Source: CAD feature listing. Evaluate the final solid. Frame: model axes, mm. A direction names the side the tool comes from. Coordinates: 2 decimals unless noted, no trailing zeros. Write each loop counter-clockwise with the first axis right and the second up, starting at its lowest first coordinate (ties: lowest second). Pieces come first, ordered by that corner, then holes. Notation, with made-up numbers: M -22.5,-23.75 L 25.5,-23.75 A34 ccw 25.5,9.25 Z; hole C 29,19 d1. An arc over 180 degrees is marked long. One line per item, written item: value. Start each with the question number.
Item 1: Set-up query: faces 1 (the flat face through (-29, 0, -7.845)), 2 (the flat face through (-3, -16.25, 11)), 3 (the flat face through (16, 27.428, 5)). Return all of +Z, -Z, +X, -X, +Y, -Y with unobstructed straight access to the full face (end or side cutting, diameter ignored); none if empty.
Item 2: Ray query, L1, parallel to X at y = -26.5, z = 9.5; L2, parallel to Y at x = -22.5, z = 8.75; L3, parallel to X at y = -12, z = 7.75. Return the intervals inside material, ascending. Write a range as from..to.
Item 3: Cut plane C-C, the plane y = 9. Output: boundary loops of the cut face in (x, z), then the cut area to 3 significant figures.
Item 4: Cut plane D-D, the plane z = -6. Output: boundary loops of the cut face in (x, y).
Item 5: Pin query (flat end, axial travel): P1, Ø5, axis at x = -8.5, z = -4.5, coming from the -Y side; P2, Ø5, axis at x = 1.5, z = -4, coming from the -Y side; P3, Ø3, axis at x = -27.5, z = -4.5, coming from the +Y side; P4, Ø1.8, axis at y = -1.5, z = -3.5, coming from the +X side. Return the tip coordinate at first contact, or that it passes through.
Item 6: Cut plane B-B, the plane z = 5.5. Output: boundary loops of the cut face in (x, y), then the cut area to 3 significant figures.
Item 7: Mould query, pull axis X, two halves, no side actions, for faces 4 (the flat face through (-28.664, -0.208, -9.431)), 5 (the flat face through (0, 27.428, -4)), 6 (the flat face through (-16, -27.928, 5)). Classes: released by +X, released by -X, zero draft, split by the parting line, or undercut.
Item 8: Cut plane A-A, the plane x = 4. Output: boundary loops of the cut face in (y, z), then the cut area to 3 significant figures.
Autodesk Inventor part; units mm, degrees
ref_plane "YZ Plane" through (0, 0, 0) normal (1, 0, 0) x (0, 1, 0)
ref_plane "XZ Plane" through (0, 0, 0) normal (0, 1, 0) x (-1, 0, 0)
ref_plane "XY Plane" through (0, 0, 0) normal (0, 0, 1) x (1, 0, 0)
sketch "Эскиз1" plane through (0, 0, 0) normal (0, 0, 1) x (1, 0, 0)
  line L0 (41.178, 40.928) -> (-41.178, 40.928) construction
  line L1 (-41.178, 40.928) -> (-41.178, -40.928) construction
  line L2 (-41.178, -40.928) -> (41.178, -40.928) construction
  line L3 (41.178, -40.928) -> (41.178, 40.928) construction
  circle A0 centre (22.7283, 19.0964) radius 1 construction
  circle A1 centre (19.3464, -22.9783) radius 1 construction
  line L4 (17.2251, 27.428) -> (22.7282, 21.9249) construction
  line L5 (22.7282, 21.9249) -> (19.8998, 19.0964) construction
  line L6 (19.8998, 19.0964) -> (22.7282, 16.268) construction
  line L7 (22.7282, 16.268) -> (25.5567, 19.0964) construction
  line L8 (25.5567, 19.0964) -> (27.678, 16.9751) construction
  line L9 (27.678, 16.9751) -> (27.678, -17.4751) construction
  line L10 (27.678, -17.4751) -> (22.1749, -22.9783) construction
  line L11 (22.1749, -22.9783) -> (19.3464, -20.1498) construction
  line L12 (19.3464, -20.1498) -> (16.518, -22.9783) construction
  line L13 (16.518, -22.9783) -> (19.3464, -25.8067) construction
  line L14 (19.3464, -25.8067) -> (17.2251, -27.928) construction
  line L15 (17.2251, -27.928) -> (-17.2251, -27.928) construction
  line L16 (-17.2251, -27.928) -> (-19.3464, -25.8067) construction
  line L17 (-19.3464, -25.8067) -> (-16.518, -22.9783) construction
  line L18 (-16.518, -22.9783) -> (-19.3464, -20.1498) construction
  line L19 (-19.3464, -20.1498) -> (-22.1749, -22.9783) construction
  line L20 (-22.1749, -22.9783) -> (-27.678, -17.4751) construction
  line L21 (-27.678, -17.4751) -> (-27.678, 16.9751) construction
  line L22 (-27.678, 16.9751) -> (-25.9871, 18.666) construction
  line L23 (-17.2251, 27.428) -> (17.2251, 27.428) construction
  line L24 (27.678, 27.428) -> (-27.678, 27.428)
  line L25 (-27.678, 27.428) -> (-27.678, -27.928)
  line L26 (-27.678, -27.928) -> (27.678, -27.928)
  line L27 (27.678, -27.928) -> (27.678, 27.428)
  line L28 (29.678, -29.928) -> (-29.678, -29.928)
  line L29 (-29.678, -29.928) -> (-29.678, 29.428)
  line L30 (-29.678, 29.428) -> (29.678, 29.428)
  line L31 (29.678, 29.428) -> (29.678, -29.928)
  circle A2 centre (-23.1587, 18.7154) radius 1
  circle A3 centre (-19.3738, -22.9783) radius 1
  line L32 (-25.9871, 18.666) -> (-23.1587, 15.8376)
  line L33 (-23.1587, 15.8376) -> (-20.3302, 18.666)
  line L34 (-20.3302, 18.666) -> (-23.1587, 21.4944)
  line L35 (-23.1587, 21.4944) -> (-17.2251, 27.428)
  point P0 (0, 0)
  dimension "d0" = 2
extrude "Выдавливание1" add sketch "Эскиз1" along normal blind 10 contours L28 L29 L30 L31
sketch "Эскиз2" plane through (0, 0, 10) normal (0, 0, 1) x (1, 0, 0)
  line L0 (29.678, 29.428) -> (-29.678, 29.428)
  line L1 (-29.678, 29.428) -> (-29.678, -29.928)
  line L2 (29.678, 29.428) -> (-29.678, 29.428)
  line L3 (-29.678, 29.428) -> (-29.678, -29.928)
  line L4 (-29.678, -29.928) -> (29.678, -29.928)
  line L5 (29.678, -29.928) -> (29.678, 29.428)
  point P0 (0, 0)
extrude "Выдавливание2" add sketch "Эскиз2" along normal blind 1.5
sketch "Эскиз3" plane through (0, 0, 10) normal (0, 0, -1) x (-1, 0, 0)
  line L0 (-27.678, 27.428) -> (-27.678, -27.928) construction
  line L1 (-27.678, -27.928) -> (27.678, -27.928) construction
  line L2 (27.678, -27.928) -> (27.678, 27.428) construction
  line L3 (27.678, 27.428) -> (-27.678, 27.428) construction
  line L4 (-29.678, -29.928) -> (-29.678, 29.428) construction
  line L5 (-29.678, -3.25) -> (-25.678, -3.25)
  line L6 (-25.678, -3.25) -> (-25.678, 2.75)
  line L7 (-25.678, 2.75) -> (-29.678, 2.75)
  line L8 (-29.678, 2.75) -> (-29.678, -3.25)
  line L9 (-27.678, 27.428) -> (-27.678, -27.928) construction
  line L10 (-27.678, -0.25) -> (27.678, -0.25) construction
  line L11 (0, -27.928) -> (0, 27.428) construction
  line L12 (29.678, -3.25) -> (25.678, -3.25)
  line L13 (25.678, -3.25) -> (25.678, 2.75)
  line L14 (25.678, 2.75) -> (29.678, 2.75)
  line L15 (29.678, 2.75) -> (29.678, -3.25)
  line L16 (-29.678, 29.428) -> (29.678, 29.428) construction
  line L17 (-3, 29.428) -> (3, 29.428)
  line L18 (3, 29.428) -> (3, 25.428)
  line L19 (3, 25.428) -> (-3, 25.428)
  line L20 (-3, 25.428) -> (-3, 29.428)
  line L21 (-3, -29.928) -> (3, -29.928)
  line L22 (3, -29.928) -> (3, -25.928)
  line L23 (3, -25.928) -> (-3, -25.928)
  line L24 (-3, -25.928) -> (-3, -29.928)
  point P0 (0, 0)
  dimension "d5" = 4
  dimension "d6" = 6
  dimension "d7" = 3
  dimension "d8" = 6
  dimension "d9" = 4
  dimension "d10" = 3
extrude "Выдавливание3" add sketch "Эскиз3" along normal blind 20
sketch "Эскиз4" plane through (0, 0, 11.5) normal (0, 0, 1) x (1, 0, 0)
  line L0 (-10, -16.25) -> (5, -16.25)
  line L1 (5, -16.25) -> (5, 15.75)
  line L2 (5, 15.75) -> (-10, 15.75)
  line L3 (-10, 15.75) -> (-10, -16.25)
  line L4 (-29.678, 29.428) -> (-29.678, -29.928) construction
  point P0 (0, 0)
  point P1 (-29.678, -0.25)
  dimension "d13" = 15
  dimension "d14" = 32
  dimension "d15" = 16
  dimension "d16" = 5
extrude "Выдавливание4" cut sketch "Эскиз4" against normal through all
sketch "Эскиз5" plane through (-3, -27.928, 10) normal (-1, 0, 0) x (0, 0, 1)
  line L0 (-20, -2) -> (-20, 2)
  line L1 (-20, 0) -> (-18.8453, -2)
  line L2 (-10, -2) -> (-20, -2)
  line L3 (-20, 0) -> (-17.6906, 0) construction
  line L4 (-18.8453, -2) -> (-17.8453, -2)
  line L5 (0, 2) -> (-20, 2)
  line L6 (-17.8453, -2) -> (-17.8453, 0)
  line L7 (-10, -2) -> (-10, 0)
  line L8 (-17.8453, 0) -> (-10, 0)
  line L9 (-10, 0) -> (-10, -2)
  line L10 (-10, -2) -> (-17.8453, -2)
  line L11 (-18.8453, -2) -> (-20, -2)
  line L12 (-20, -2) -> (-20, 0)
  point P0 (-10, 27.928)
  point P1 (-17.8453, -2)
  dimension "d19" = 60
  dimension "d20" = 1
extrude "Выдавливание5" cut sketch "Эскиз5" against normal up to surface (6 mm away)
sketch "Эскиз6" plane through (-3, 25.428, 10) normal (-1, 0, 0) x (0, 0, 1)
  line L0 (-20, 4) -> (-20, 0)
  line L1 (-20, 2) -> (-18.8453, 4)
  line L2 (-10, 4) -> (-20, 4)
  line L3 (-20, 2) -> (-17.6906, 2) construction
  line L4 (-10, 4) -> (1.5, 4)
  line L5 (-17.8453, 4) -> (-10, 4)
  line L6 (-10, 4) -> (-10, 2)
  line L7 (-10, -22.678) -> (-10, 4)
  line L8 (-17.8453, 2) -> (-17.8453, 4)
  line L9 (-17.8453, 2) -> (-10, 2)
  line L10 (-10, 2) -> (-10, 4)
  line L11 (-20, 2) -> (-20, 4)
  line L12 (-18.8453, 4) -> (-20, 4)
  point P0 (-10, -25.428)
  dimension "d23" = 60
extrude "Выдавливание6" cut sketch "Эскиз6" against normal up to surface (6 mm away)
sketch "Эскиз7" plane through (25.678, 2.75, 10) normal (0, 1, 0) x (1, 0, 0)
  line L0 (4, 20) -> (0, 20)
  line L1 (2, 20) -> (4, 18.8453)
  line L2 (4, 10) -> (4, 20)
  line L3 (2, 20) -> (4.3094, 20) construction
  line L4 (4, 18.8453) -> (4, 20)
  line L5 (0, 20) -> (4, 20)
  line L6 (4, 20) -> (2, 20)
  line L7 (4, 17.8453) -> (2, 17.8453)
  line L8 (2, 10) -> (2, 0)
  line L9 (2, 17.8453) -> (2, 10)
  line L10 (-55.356, 10) -> (4, 10)
  line L11 (2, 10) -> (4, 10)
  line L12 (-22.678, 10) -> (2, 10)
  line L13 (4, 10) -> (2, 10)
  line L14 (4, 10) -> (4, 17.8453)
  point P0 (-25.678, 10)
  dimension "d27" = 30
extrude "Выдавливание7" cut sketch "Эскиз7" against normal up to surface (6 mm away)
sketch "Эскиз8" plane through (-27.678, 2.75, 10) normal (0, 1, 0) x (1, 0, 0)
  line L0 (-2, 20) -> (2, 20)
  line L1 (0, 20) -> (-2, 20)
  line L2 (0, 20) -> (-2, 18.8453)
  line L3 (-2, 10) -> (-2, 20)
  line L4 (0, 20) -> (2.3094, 20) construction
  line L5 (-2, 17.8453) -> (0, 17.8453)
  line L6 (0, 10) -> (0, 0)
  line L7 (0, 17.8453) -> (0, 10)
  line L8 (-2, 10) -> (57.356, 10)
  line L9 (0, 10) -> (-2, 10)
  line L10 (-2, 10) -> (-2, 17.8453)
  line L11 (-2, 18.8453) -> (-2, 20)
  point P0 (27.678, 10)
  dimension "d31" = 150
extrude "Выдавливание8" cut sketch "Эскиз8" against normal up to surface (6 mm away)
properties part number "Верх"
From the geometry:
1. face 1: -X, +Y, -Y
1. face 2: +Z, -Z
1. face 3: -Z
2. L1: x = -29.68..-27.68, -3..3, 27.68..29.68
2. L2: y = -29.93..-27.93, 27.43..29.43
2. L3: x = -29.68..-27.68, 27.68..29.68
3. outline: M -29.68,0 L -27.68,0 L -27.68,10 L -10,10 L -10,11.5 L -29.68,11.5 Z; M 5,10 L 27.68,10 L 27.68,0 L 29.68,0 L 29.68,11.5 L 5,11.5 Z
3. area: 107 mm²
4. outline: M -27.68,-3.25 L -25.68,-3.25 L -25.68,2.75 L -27.68,2.75 Z; M -3,-27.93 L 3,-27.93 L 3,-25.93 L -3,-25.93 Z; M -3,25.43 L 3,25.43 L 3,27.43 L -3,27.43 Z; M 25.68,-3.25 L 27.68,-3.25 L 27.68,2.75 L 25.68,2.75 Z
5. P1: passes through
5. P2: stops at y = -27.93
5. P3: stops at y = 2.75
5. P4: stops at x = 27.68
6. outline: M -29.68,-29.93 L 29.68,-29.93 L 29.68,29.43 L -29.68,29.43 Z; hole M -27.68,-27.93 L -3,-27.93 L -3,-25.93 L 3,-25.93 L 3,-27.93 L 27.68,-27.93 L 27.68,-3.25 L 25.68,-3.25 L 25.68,2.75 L 27.68,2.75 L 27.68,27.43 L 3,27.43 L 3,25.43 L -3,25.43 L -3,27.43 L -27.68,27.43 L -27.68,2.75 L -25.68,2.75 L -25.68,-3.25 L -27.68,-3.25 Z
6. area: 507 mm²
7. face 4: released by -X
7. face 5: zero draft
7. face 6: undercut
8. outline: M -29.93,0 L -27.93,0 L -27.93,10 L -16.25,10 L -16.25,11.5 L -29.93,11.5 Z; M 15.75,10 L 27.43,10 L 27.43,0 L 29.43,0 L 29.43,11.5 L 15.75,11.5 Z
8. area: 81.0 mm²
